Geometry check sheet. Reference: drawing and pictorial views, mm from the part's lowest x, y, z. A direction names the side the tool comes from. Coordinates: 2 decimals unless noted, no trailing zeros. Write each loop counter-clockwise with the first axis right and the second up, starting at its lowest first coordinate (ties: lowest second). Pieces come first, ordered by that corner, then holes. Notation, with made-up numbers: (19, 57) -> (45, 57) arc R27 cw to (45, 89) -> close; hole circle Ø10 at (77.25, 24.5). An arc over 180 degrees is marked (long way). Put each result on its own line as item: value.
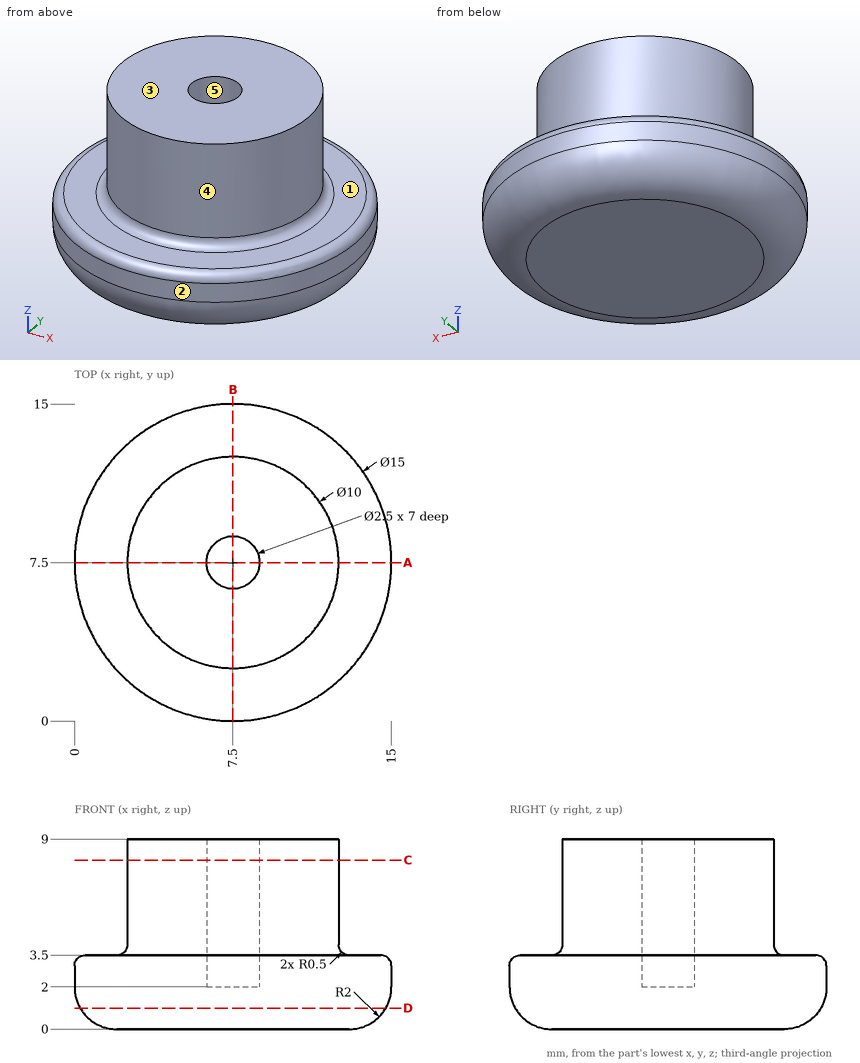
Q1. Material ranges on line 1 along Y through (x, z) = (7.5, 4.25); line 2 along X through (y, z) = (8.5, 2.25); line 3 along X through (y, z) = (6.5, 4.75), recorded low to high.
Recorded:
line 1: y = 2.5 to 6.25, 8.75 to 12.5
line 2: x = 0.07 to 6.75, 8.25 to 14.93
line 3: x = 2.6 to 6.75, 8.25 to 12.4
Q2. Cross-section at C-C (z = 8). Record the cut outline in (x, y), plus the area to 3 significant figures.
Recorded:
outline: circle Ø10 at (7.5, 7.5); hole circle Ø2.5 at (7.5, 7.5)
area: 73.6 mm2
Q3. Cross-section at A-A (y = 7.5). Record the cut outline in (x, z), plus the area to 3 significant figures.
Recorded:
outline: (0, 2) arc R2 ccw to (2, 0) -> (13, 0) arc R2 ccw to (15, 2) -> (15, 3) arc R0.5 ccw to (14.5, 3.5) -> (13, 3.5) arc R0.5 cw to (12.5, 4) -> (12.5, 9) -> (8.75, 9) -> (8.75, 2) -> (6.25, 2) -> (6.25, 9) -> (2.5, 9) -> (2.5, 4) arc R0.5 cw to (2, 3.5) -> (0.5, 3.5) arc R0.5 ccw to (0, 3) -> close
area: 88.3 mm2
Q4. Tool access check on the marked faces 1 and 2. Record the directions out of +Z, -Z, +X, -X, +Y, -Y that give a thin tool (end or side, any length) a straight path to the whole face; none if there is none.
Recorded:
face 1: +Z
face 2: +Z, -Z
Q5. Depth check by flat-ended pin: P1, Ø0.8, axis at x = 7, y = 7.5, coming from the +Z side; P2, Ø5, axis at x = 8.5, z = 7.5, coming from the -Y side; P3, Ø4, axis at x = 10.5, z = 3, coming from the -Y side. Enter the tip coordinate at first touch or a pass-through.
Recorded:
P1: stops at z = 2
P2: stops at y = 2.5
P3: stops at y = 0.07
Q6. Mould release check, pull along X, two halves, no side actions. Record for the marked faces 3, 4 and 5: released by +X, released by -X, zero draft, split by the parting line, or undercut.
Recorded:
face 3: zero draft
face 4: split by the parting line
face 5: undercut
Q7. Cross-section at D-D (z = 1). Record the cut outline in (x, y), plus the area to 3 significant figures.
Recorded:
outline: circle Ø14.46 at (7.5, 7.5)
area: 164 mm2
